For this review, use the dimensioned drawing (mm, ordinates from the lowest corner) and the shaded views. A direction names the side the tool comes from. Round coordinates to 2 decimals unless told otherwise and drop trailing zeros. Order: outer loops, then holes, each group sorted by start corner. A loop starts at its lowest first (then second) coordinate and runs counter-clockwise, first axis right, second up. Notation, with made-up numbers: M -9,-38 L 49,-38 A28 cw 49,-7 Z; hole C -1,87.25 d6. An arc over 180 degrees is marked long. One line per item, written item: value. Start each with the question number.
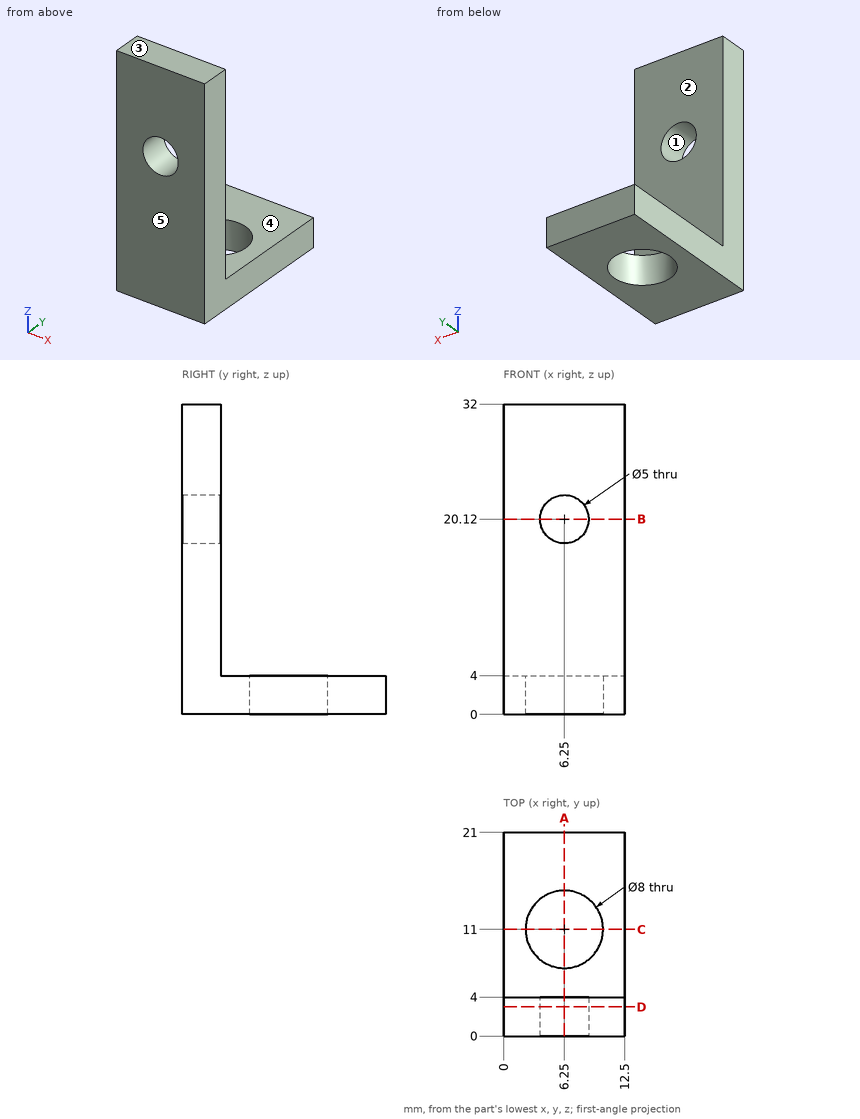
Item 1: Machinability: for the marked faces 4 and 5, which of the approach directions +Z, -Z, +X, -X, +Y, -Y give a long, thin tool a straight path to every point of the face, cutting with its end or side? Answer none if there is none.
Item 2: Consider section A-A, the plane x = 6.25. Give the boundary of the cut face in (y, z), then the cut area to 3 significant figures.
Item 3: Clearance check with flat-ended pins moving along their axes: P1, Ø3, axis at y = 11, z = 6.5, coming from the -X side; P2, Ø2, axis at x = 9.5, z = 20, coming from the +Y side. State where each tip first meets the part, or that it passes through.
Item 4: Wall thickness on L1, parallel to X at y = 2, z = 20.12; L2, parallel to Y at x = 7.5, z = 12: over which ranges is each line inside the solid? List them lowest first.
Item 5: The part is to be moulded in two halves that separate along Z. For the marked faces 1, 2 and 3, say which applies: pulls with the +Z half, pulls with the -Z half, needs draft (parallel to the pull), parting line crosses it, or undercut.
Item 6: Consider section D-D, the plane y = 3. Give the boundary of the cut face in (x, z), then the cut area to 3 significant figures.
Item 7: Consider section C-C, the plane y = 11. Give the boundary of the cut face in (x, z).
Item 8: Consider section B-B, the plane z = 20.12. Give the boundary of the cut face in (x, y), then the cut area to 3 significant figures.
Computed:
1. face 4: +Z, +X, -X, +Y
1. face 5: +Z, -Z, +X, -X, -Y
2. outline: M 0,0 L 7,0 L 7,4 L 4,4 L 4,17.62 L 0,17.62 Z; M 0,22.62 L 4,22.62 L 4,32 L 0,32 Z; M 15,0 L 21,0 L 21,4 L 15,4 Z
2. area: 144 mm^2
3. P1: passes through
3. P2: stops at y = 4
4. L1: x = 0 to 3.75, 8.75 to 12.5
4. L2: y = 0 to 4
5. face 1: undercut
5. face 2: needs draft
5. face 3: pulls with the +Z half
6. outline: M 0,0 L 12.5,0 L 12.5,32 L 0,32 Z; hole C 6.25,20.12 d5
6. area: 380 mm^2
7. outline: M 0,0 L 2.25,0 L 2.25,4 L 0,4 Z; M 10.25,0 L 12.5,0 L 12.5,4 L 10.25,4 Z
8. outline: M 0,0 L 3.75,0 L 3.75,4 L 0,4 Z; M 8.75,0 L 12.5,0 L 12.5,4 L 8.75,4 Z
8. area: 30.0 mm^2
